Geometry: final body of the model. Coordinates: model frame, mm. A direction names the side the tool comes from. Give positions to 0.01 mm unless a question says otherwise; leave off trailing zeros. Order: outer loops, then holes, each group sorted by start corner. A loop starts at its lowest first (then second) coordinate and runs counter-clockwise, first axis right, second up. Notation, with made-up numbers: M 45.5,6.5 L 80.5,6.5 A21 cw 80.5,40.5 Z; hole C 36,16 d10. An arc over 180 degrees is marked long. Write item = value, one per line. Start each with the question number.
from build123d import *

# Parameters (mm, degrees)
SKETCH1_W           = 28.8417
SKETCH1_H           = 2.8575
BOSS_EXTRUDE1_DEPTH = 28.575


with BuildPart() as part:
    # Sketch1 → Boss-Extrude1 (new body)
    with BuildSketch(Plane(origin=(0, 0, 0), x_dir=(0, 0, -1), z_dir=(1, 0, 0))):
        with Locations((14.42085, 4.60375)):
            Rectangle(SKETCH1_W, SKETCH1_H)
        with BuildLine():
            ThreePointArc((0, 2.032), (-2.032, 0), (0, -2.032))
            Line((0, -2.032), (0, -6.0325))
            ThreePointArc((0, -6.0325), (-6.0325, 0), (0, 6.0325))
            Line((0, 6.0325), (0, 2.032))
        make_face()
        with Locations((14.42085, -4.60375)):
            Rectangle(SKETCH1_W, SKETCH1_H)
    extrude(amount=BOSS_EXTRUDE1_DEPTH)


solid = part.part
1) Cut plane C-C (y = 0). Return loops of the section in (x, z) (1 decimal), plus the area to 3 significant figures.
2) Access query for faces 1 (the flat face through (14, 3, 0)), 2 (the flat face through (14, -5, -28.842)). Directions: +Z, -Z, +X, -X, +Y, -Y. A direction counts if a zero-diameter tool reaches every point of the face in a straight line with its end or side. Return the directions, or none.
3) Cut plane B-B (x = 21.25). Return loops of the section in (y, z) (1 decimal).
4) Draft query along Y for faces 3 (the flat face through (14, -3, 0)), 4 (the flat face through (0, 4, -11)), 5 (the flat face through (14, 6.032, -14)), 6 (the flat face through (14, 3.175, -14)). Return one class per face: pulls with the +Y half, pulls with the -Y half, needs draft (parallel to the pull), parting line crosses it, or undercut.
5) Cut plane A-A (z = -23). Return loops of the section in (x, y) (1 decimal).
6) Cut plane D-D (z = 0.5). Return loops of the section in (x, y) (3 decimals), plus the area to 3 significant figures.
7) Ray query, L1, parallel to Y at x = 25.25, z = -8.5 (1 decimal); L2, parallel to Z at x = 1.75, y = 0; L3, parallel to Y at x = 25.5, z = 0.5. Return the intervals inside material, ascending.
8) Pin query (flat end, axial travel): pin 1 Ø1 at (x, y) = (8.5, 2.5) entering from -Z; pin 2 Ø2 at (y, z) = (-1, -12.5) entering from -X; pin 3 Ø1 at (x, y) = (14, 3) entering from +Z. Return the tip coordinate at first contact, or that it passes through.
Reply:
q1.outline = M 0,2 L 28.6,2 L 28.6,6 L 0,6 Z
q1.area = 114 mm²
q2.face_1 = -Z, +X, -X
q2.face_2 = -Z, +X, -X, +Y, -Y
q3.outline = M -6,-28.8 L -3.2,-28.8 L -3.2,0 L -2,0 A2 cw 2,0 L 3.2,0 L 3.2,-28.8 L 6,-28.8 L 6,0 A6 ccw -6,0 Z
q4.face_3 = undercut
q4.face_4 = needs draft
q4.face_5 = pulls with the +Y half
q4.face_6 = undercut
q5.outline = M 0,-6 L 28.6,-6 L 28.6,-3.2 L 0,-3.2 Z; M 0,3.2 L 28.6,3.2 L 28.6,6 L 0,6 Z
q6.outline = M 0,-6.012 L 28.575,-6.012 L 28.575,-1.97 L 0,-1.97 Z; M 0,1.97 L 28.575,1.97 L 28.575,6.012 L 0,6.012 Z
q6.area = 231 mm²
q7.L1 = -6 to -3.2, 3.2 to 6
q7.L2 = 2.03 to 6.03
q7.L3 = -6.01 to -1.97, 1.97 to 6.01
q8.pin_1 = 0
q8.pin_2 = through
q8.pin_3 = 5.49
